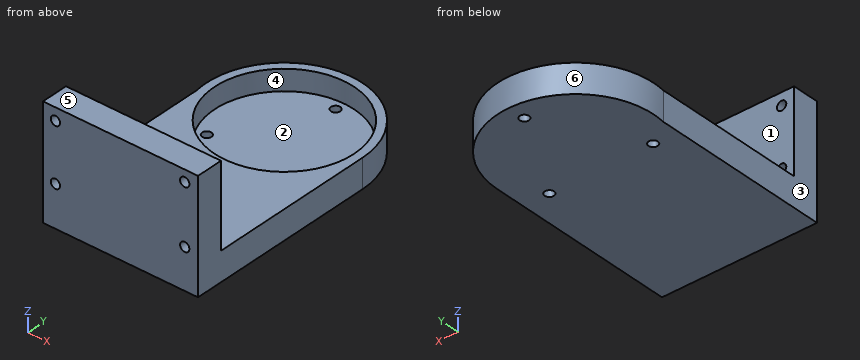
Autodesk Inventor part; units mm, degrees
ref_plane "YZ Plane" through (0, 0, 0) normal (1, 0, 0) x (0, 1, 0)
ref_plane "XZ Plane" through (0, 0, 0) normal (0, 1, 0) x (-1, 0, 0)
ref_plane "XY Plane" through (0, 0, 0) normal (0, 0, 1) x (1, 0, 0)
sketch "草图1" plane through (0, 0, 0) normal (0, 0, 1) x (1, 0, 0)
  circle A0 centre (0, 0) radius 33.75
  circle A1 centre (0, 0) radius 29
  circle A2 centre (0, 29) radius 2.25
  circle A3 centre (-25.1147, -14.5) radius 2.25
  circle A4 centre (25.1147, -14.5) radius 2.25
  circle A5 centre (0, 0) radius 37.75
  circle A6 centre (0, 0) radius 23.5
  dimension "d1" = 58
  dimension "d0" = 67.5
  dimension "d2" = 4.5
  dimension "d5" = 360
  dimension "d7" = 4
  dimension "d13" = 47
sketch "草图2" plane through (0, 0, 0) normal (0, 1, 0) x (-1, 0, 0)
  line L0 (37.75, 0) -> (-37.75, 0)
  line L1 (-37.75, 0) -> (37.25, 0)
  line L2 (37.25, 0) -> (37.25, 10)
  line L3 (37.25, 10) -> (-37.75, 10)
  line L4 (-37.75, 10) -> (-37.75, 0)
  line L5 (37.25, 0) -> (-37.75, 0)
  line L6 (-37.75, 0) -> (-37.75, -4)
  line L7 (-37.75, -4) -> (37.25, -4)
  line L8 (37.25, -4) -> (37.25, 0)
  point P0 (0, 0)
  dimension "d8" = 75
  dimension "d9" = 10
  dimension "d12" = 4
extrude "拉伸1" add sketch "草图2" against normal blind 80
extrude "拉伸2" cut sketch "草图1" along normal blind 10 contours A0 | A1 A4 A3 A2 | A2 A1 | A1 A2 | A4 A1 | A1 A4 | A3 A1 | A1 A3 | A6
extrude "拉伸3" cut sketch "草图1" against normal blind 10 contours A2 A1 | A1 A2 | A4 A1 | A1 A4 | A3 A1 | A1 A3
extrude "拉伸4" add sketch "草图1" against normal blind 4 contours A0 | A1 A4 A3 A2 | A5 | A6
extrude "拉伸5" add sketch "草图1" along normal blind 10 contours A5
sketch "草图3" plane through (0, -80, 0) normal (0, -1, 0) x (1, 0, 0)
  line L0 (-37.25, 10) -> (-37.25, -4)
  line L1 (-37.25, -4) -> (37.75, -4)
  line L2 (37.75, -4) -> (37.75, 10)
  line L3 (37.75, 10) -> (-37.25, 10)
  line L4 (37.75, 0) -> (-37.25, 0)
  line L5 (-37.25, 0) -> (-37.25, 50)
  line L6 (-37.25, 50) -> (37.75, 50)
  line L7 (37.75, 50) -> (37.75, 0)
  line L8 (37.75, -4) -> (-37.25, -4)
  line L9 (-37.25, -4) -> (-37.25, 0)
  line L10 (-37.25, 0) -> (37.75, 0)
  line L11 (37.75, 0) -> (37.75, -4)
  circle A0 centre (-31.25, 44) radius 2.25
  line L12 (0.25, 10) -> (0, 50)
  circle A1 centre (31.3226, 44.3911) radius 2.25
  line L13 (-37.25, 30) -> (37.75, 30)
  circle A2 centre (-31.25, 16) radius 2.25
  circle A3 centre (31.3226, 15.6089) radius 2.25
  point P0 (0, 0)
  dimension "d22" = 50
  dimension "d25" = 4.5
  dimension "d26" = 6
  dimension "d27" = 6
extrude "拉伸6" add sketch "草图3" along normal blind 13
properties part number "电机支架-v0.1.0"
Here's how the part is built. I have some questions about the finished solid (model axes, mm). Face numbers are marked on the shaded views. A direction names the side the tool comes from. Round coordinates to 2 decimals unless told otherwise and drop trailing zeros. Write each loop counter-clockwise with the first axis right and the second up, starting at its lowest first coordinate (ties: lowest second). Pieces come first, ordered by that corner, then holes.
1. Suppose I cut it at A-A (x = 0). List the corners of the cut face in (y, z) for me, and give its area (3 significant figures).
2. Suppose I cut it at C-C (z = 2). List the corners of the cut face in (x, y) for me.
3. Will these pins go through, and if not, where does the flat tip stop? pin 1 Ø10 at (x, z) = (-2.5, 28) entering from +Y; pin 2 Ø10 at (x, y) = (15, 8) entering from +Z; pin 3 Ø22.5 at (x, y) = (-8.5, -48.5) entering from +Z.
4. Suppose I cut it at B-B (y = -14.5). List the corners of the cut face in (x, z) for me.
5. I need wall thicknesses on L1, parallel to Z at x = -31.25, y = -85.25; L2, parallel to X at y = -14.5, z = -3.05; L3, parallel to Y at x = 32, z = 19. Which ranges of each line are inside material? Lowest first, please.
6. For the marked faces 1, 2 and 3, which set-ups out of +Z, -Z, +X, -X, +Y, -Y let a thin tool reach every point of the face, with its end or its side?
7. If we mould it in two halves opening along X, with no side actions, what happens to the marked faces 4, 5 and 6? For each: released by +X, released by -X, zero draft, split by the parting line, or undercut.
8. Suppose I cut it at D-D (y = 29). List the corners of the cut face in (x, z) for me, and give its area (3 significant figures).
Answer sheet:
1. outline: (-93, -4) - (26.75, -4) - (26.75, 0) - (-33.75, 0) - (-33.75, 10) - (-80, 10) - (-80, 50) - (-93, 50) - close; (31.25, -4) - (37.75, -4) - (37.75, 10) - (33.75, 10) - (33.75, 0) - (31.25, 0) - close
1. area: 1,660 mm2
2. outline: (-37.25, -93) - (37.75, -93) - (37.75, 0) arc R37.75 ccw (long way) to (-37.25, -6.12) - close; hole circle Ø67.5 at (0, 0)
3. pin 1: stops at y = -80
3. pin 2: stops at z = 0
3. pin 3: stops at z = 10
4. outline: (-37.25, -4) - (-27.36, -4) - (-27.36, 0) - (-30.48, 0) - (-30.48, 10) - (-37.25, 10) - close; (-22.86, -4) - (22.86, -4) - (22.86, 0) - (-22.86, 0) - close; (27.36, -4) - (37.75, -4) - (37.75, 10) - (30.48, 10) - (30.48, 0) - (27.36, 0) - close
5. L1: z = -4 to 13.75, 18.25 to 41.75, 46.25 to 50
5. L2: x = -37.25 to -27.36, -22.86 to 22.86, 27.36 to 37.75
5. L3: y = -93 to -80
6. face 1: +Z, +X, -X, +Y
6. face 2: +Z
6. face 3: +Z, -Z, -X, -Y
7. face 4: undercut
7. face 5: zero draft
7. face 6: split by the parting line
8. outline: (-24.17, -4) - (-2.25, -4) - (-2.25, 0) - (-17.26, 0) - (-17.26, 10) - (-24.17, 10) - close; (2.25, -4) - (24.17, -4) - (24.17, 10) - (17.26, 10) - (17.26, 0) - (2.25, 0) - close
8. area: 313 mm2
